from build123d import *

# Parameters (mm, degrees)
SKETCH_1_W          = 76
SKETCH_1_H          = 60
EXTRUDE_1_DEPTH     = 2
EXTRUDE_2_DEPTH     = 3.35
SKETCH_2_W          = 76
SKETCH_2_H          = 60
CUT_EXTRUDE_1_DEPTH = 2.95
SKETCH_3_R          = 2.55
CUT_EXTRUDE_2_DEPTH = 45.193605611
SKETCH_4_R          = 7.5
CUT_EXTRUDE_3_DEPTH = 45.193605611
SKETCH_5_R          = 1.5
CUT_EXTRUDE_4_DEPTH = 45.193605611
SKETCH_6_R          = 2.5
CUT_EXTRUDE_5_DEPTH = 45.193605611
CUT_EXTRUDE_6_DEPTH = 4
CUT_EXTRUDE_7_DEPTH = 4
CUT_EXTRUDE_8_DEPTH = 4


with BuildPart() as part:
    # 草圖1 → 填料-伸長1 (new body)
    with BuildSketch(Plane.XY):
        Rectangle(SKETCH_1_W, SKETCH_1_H)
        with BuildLine():
            ThreePointArc((-6.225922266, -9.22263808), (-5.992959353, -9.526241259), (-6.042909564, -9.905650781))
            Line((-6.042909564, -9.905650781), (-7.592909564, -12.590329533))
            ThreePointArc((-7.592909564, -12.590329533), (-7.896512744, -12.823292446), (-8.275922266, -12.773342235))
            Line((-8.275922266, -12.773342235), (-10.007973074, -11.773342235))
            ThreePointArc((-10.007973074, -11.773342235), (-10.240935987, -11.469739056), (-10.190985776, -11.090329533))
            Line((-10.190985776, -11.090329533), (-8.640985776, -8.405650781))
            ThreePointArc((-8.640985776, -8.405650781), (-8.337382596, -8.172687868), (-7.957973074, -8.22263808))
            Line((-7.957973074, -8.22263808), (-6.225922266, -9.22263808))
        make_face(mode=Mode.SUBTRACT)
        with BuildLine():
            Line((-12.313100093, -5.76593935), (-14.313100093, -9.230040965))
            ThreePointArc((-14.313100093, -9.230040965), (-14.996112795, -9.413053667), (-15.179125497, -8.730040965))
            Line((-15.179125497, -8.730040965), (-13.179125497, -5.26593935))
            ThreePointArc((-13.179125497, -5.26593935), (-12.496112795, -5.082926648), (-12.313100093, -5.76593935))
        make_face(mode=Mode.SUBTRACT)
        with BuildLine():
            ThreePointArc((11.15, -8.780487805), (10.65, -8.280487805), (11.15, -7.780487805))
            Line((11.15, -7.780487805), (15.15, -7.780487805))
            ThreePointArc((15.15, -7.780487805), (15.65, -8.280487805), (15.15, -8.780487805))
            Line((15.15, -8.780487805), (11.15, -8.780487805))
        make_face(mode=Mode.SUBTRACT)
        with BuildLine():
            Line((-5.557090436, 10.186138586), (-7.107090436, 12.870817338))
            ThreePointArc((-7.107090436, 12.870817338), (-7.157040647, 13.250226861), (-6.924077734, 13.55383004))
            Line((-6.924077734, 13.55383004), (-5.192026926, 14.55383004))
            ThreePointArc((-5.192026926, 14.55383004), (-4.812617404, 14.603780251), (-4.509014224, 14.370817338))
            Line((-4.509014224, 14.370817338), (-2.959014224, 11.686138586))
            ThreePointArc((-2.959014224, 11.686138586), (-2.909064013, 11.306729064), (-3.142026926, 11.003125884))
            Line((-3.142026926, 11.003125884), (-4.874077734, 10.003125884))
            ThreePointArc((-4.874077734, 10.003125884), (-5.253487256, 9.953175673), (-5.557090436, 10.186138586))
        make_face(mode=Mode.SUBTRACT)
        with BuildLine():
            Line((1.163100093, 13.546427155), (-0.836899907, 17.01052877))
            ThreePointArc((-0.836899907, 17.01052877), (-0.653887205, 17.693541472), (0.029125497, 17.51052877))
            Line((0.029125497, 17.51052877), (2.029125497, 14.046427155))
            ThreePointArc((2.029125497, 14.046427155), (1.846112795, 13.363414453), (1.163100093, 13.546427155))
        make_face(mode=Mode.SUBTRACT)
    extrude(amount=EXTRUDE_1_DEPTH)

    # 草圖1<3> → 填料-伸長2 (add)
    with BuildSketch(Plane.XY):
        with BuildLine():
            Line((14.7, -0.280487805), (11.6, -0.280487805))
            ThreePointArc((11.6, -0.280487805), (11.246446609, -0.426934414), (11.1, -0.780487805))
            Line((11.1, -0.780487805), (11.1, -2.780487805))
            ThreePointArc((11.1, -2.780487805), (11.246446609, -3.134041195), (11.6, -3.280487805))
            Line((11.6, -3.280487805), (14.7, -3.280487805))
            ThreePointArc((14.7, -3.280487805), (15.053553391, -3.134041195), (15.2, -2.780487805))
            Line((15.2, -2.780487805), (15.2, -0.780487805))
            ThreePointArc((15.2, -0.780487805), (15.053553391, -0.426934414), (14.7, -0.280487805))
        make_face()
        with BuildLine():
            Line((-7.107090436, 12.870817338), (-5.557090436, 10.186138586))
            ThreePointArc((-5.557090436, 10.186138586), (-5.253487256, 9.953175673), (-4.874077734, 10.003125884))
            Line((-4.874077734, 10.003125884), (-3.142026926, 11.003125884))
            ThreePointArc((-3.142026926, 11.003125884), (-2.909064013, 11.306729064), (-2.959014224, 11.686138586))
            Line((-2.959014224, 11.686138586), (-4.509014224, 14.370817338))
            ThreePointArc((-4.509014224, 14.370817338), (-4.812617404, 14.603780251), (-5.192026926, 14.55383004))
            Line((-5.192026926, 14.55383004), (-6.924077734, 13.55383004))
            ThreePointArc((-6.924077734, 13.55383004), (-7.157040647, 13.250226861), (-7.107090436, 12.870817338))
        make_face()
        with BuildLine():
            Line((-6.042909564, -9.905650781), (-7.592909564, -12.590329533))
            ThreePointArc((-7.592909564, -12.590329533), (-7.896512744, -12.823292446), (-8.275922266, -12.773342235))
            Line((-8.275922266, -12.773342235), (-10.007973074, -11.773342235))
            ThreePointArc((-10.007973074, -11.773342235), (-10.240935987, -11.469739056), (-10.190985776, -11.090329533))
            Line((-10.190985776, -11.090329533), (-8.640985776, -8.405650781))
            ThreePointArc((-8.640985776, -8.405650781), (-8.337382596, -8.172687868), (-7.957973074, -8.22263808))
            Line((-7.957973074, -8.22263808), (-6.225922266, -9.22263808))
            ThreePointArc((-6.225922266, -9.22263808), (-5.992959353, -9.526241259), (-6.042909564, -9.905650781))
        make_face()
    extrude(amount=EXTRUDE_2_DEPTH)

    # 草圖2 → 除料-伸長1 (cut)
    with BuildSketch(Plane(origin=(0, 0, 0), x_dir=(-1, 0, 0), z_dir=(0, 0, -1))):
        Rectangle(SKETCH_2_W, SKETCH_2_H)
        with BuildLine():
            ThreePointArc((-29.9, 26.904317068), (-33.435533906, 25.439850974), (-34.9, 21.904317068))
            Line((-34.9, 21.904317068), (-34.9, -21.9))
            ThreePointArc((-34.9, -21.9), (-33.435533906, -25.435533906), (-29.9, -26.9))
            Line((-29.9, -26.9), (29.9, -26.9))
            ThreePointArc((29.9, -26.9), (33.435533906, -25.435533906), (34.9, -21.9))
            Line((34.9, -21.9), (34.9, 21.904317068))
            ThreePointArc((34.9, 21.904317068), (33.435533906, 25.439850974), (29.9, 26.904317068))
            Line((29.9, 26.904317068), (-29.9, 26.904317068))
        make_face(mode=Mode.SUBTRACT)
    extrude(amount=-CUT_EXTRUDE_1_DEPTH, mode=Mode.SUBTRACT)

    # 草圖3 → 除料-伸長2 (cut, through all)
    with BuildSketch(Plane(origin=(0, 0, 0), x_dir=(-1, 0, 0), z_dir=(0, 0, -1))):
        with Locations((20.5, 0)):
            Circle(SKETCH_3_R)
        with Locations((-20.5, 0)):
            Circle(SKETCH_3_R)
        with Locations((-10.25, -17.753520778)):
            Circle(SKETCH_3_R)
        with Locations((-10.25, 17.753520778)):
            Circle(SKETCH_3_R)
        with Locations((10.25, 17.753520778)):
            Circle(SKETCH_3_R)
        with Locations((10.25, -17.753520778)):
            Circle(SKETCH_3_R)
    extrude(amount=-CUT_EXTRUDE_2_DEPTH, mode=Mode.SUBTRACT)

    # 草圖4 → 除料-伸長3 (cut, through all)
    with BuildSketch(Plane(origin=(0, 0, 0), x_dir=(-1, 0, 0), z_dir=(0, 0, -1))):
        Circle(SKETCH_4_R)
    extrude(amount=-CUT_EXTRUDE_3_DEPTH, mode=Mode.SUBTRACT)

    # 草圖5 → 除料-伸長4 (cut, through all)
    with BuildSketch(Plane(origin=(0, 0, 0), x_dir=(-1, 0, 0), z_dir=(0, 0, -1))):
        with Locations((-32.4, 19.404317068)):
            Circle(SKETCH_5_R)
        with Locations(Location((-32.402400032, -19.400309097, 0), (0, 0, 180))):
            Circle(SKETCH_5_R)
        with Locations((32.402400032, -19.400309097)):
            Circle(SKETCH_5_R)
        with Locations((32.402400032, 17.904317068)):
            Circle(SKETCH_5_R)
    extrude(amount=-CUT_EXTRUDE_4_DEPTH, mode=Mode.SUBTRACT)

    # 草圖6 → 除料-伸長5 (cut, through all)
    with BuildSketch(Plane(origin=(0, 0, 0), x_dir=(-1, 0, 0), z_dir=(0, 0, -1))):
        with Locations((-21.9, 16.904317068)):
            Circle(SKETCH_6_R)
        with Locations(Location((21.9, 16.904317068, 0), (0, 0, 180))):
            Circle(SKETCH_6_R)
        with Locations((-21.9, -19.4)):
            Circle(SKETCH_6_R)
    extrude(amount=-CUT_EXTRUDE_5_DEPTH, mode=Mode.SUBTRACT)

    # 草圖7 → 除料-伸長6 (cut)
    with BuildSketch(Plane.ZY.offset(-11.15)):
        Polygon((2, -8.780487805), (0, -8.780487805), (0, -13.780487805), (2, -11.780487805), align=None)
    extrude(amount=-CUT_EXTRUDE_6_DEPTH, mode=Mode.SUBTRACT)

    # 草圖8 → 除料-伸長7 (cut)
    with BuildSketch(Plane(origin=(-5.575, 9.656183252, 0), x_dir=(-0.8660254037844417, -0.4999999999999947, 0), z_dir=(0.49999999999999484, -0.8660254037844418, 0))):
        Polygon((-8.780487805, -2), (-8.780487805, 0), (-13.780487805, 0), (-11.780487805, -2), align=None)
    extrude(amount=-CUT_EXTRUDE_7_DEPTH, mode=Mode.SUBTRACT)

    # 草圖9 → 除料-伸長8 (cut)
    with BuildSketch(Plane(origin=(-5.575, -9.656183252, 0), x_dir=(0.8660254037844359, -0.5000000000000049, 0), z_dir=(0.5000000000000048, 0.8660254037844358, 0))):
        Polygon((-8.780487805, -2), (-8.780487805, 0), (-13.780487805, 0), (-11.780487805, -2), align=None)
    extrude(amount=-CUT_EXTRUDE_8_DEPTH, mode=Mode.SUBTRACT)


solid = part.part
For this review, take the finished solid that the model builds, in its own axes (mm). A direction names the side the tool comes from. Coordinates: 2 decimals unless noted, no trailing zeros. Loops run counter-clockwise (first coordinate to the right, second up) from the corner with the lowest first, then second, coordinate; pieces in that order, holes last. Notation, with made-up numbers: (17.25, 49) - (44.25, 49) arc R28 cw to (44.25, 72) - close; hole circle Ø2 at (58, -25). An arc over 180 degrees is marked (long way). Return JSON: item names as keys, results as strings.
Item 1: For faces 1 (the flat face through (-3.723, 13.01, 2.666)), 2 (the flat face through (13.12, -12.79, 0.99)), 3 (the flat face through (-6.807, -11.229, 2.666)), list the 3-axis set-ups (+Z, -Z, +X, -X, +Y, -Y) from which the entire face can be reached by the end or side of a thin tool; tool diameter is ignored.
Determined:
{"face 1": "+Z, +X, +Y", "face 2": "-Z", "face 3": "+Z, +X, -Y"}
Item 2: Take a section at C-C (x = -21.9). Give the boundary of the cut face in (y, z).
Determined:
{"outline": "(-26.9, 0) - (-2.13, 0) - (-2.13, 2) - (-26.9, 2) - close; (2.13, 0) - (14.4, 0) - (14.4, 2) - (2.13, 2) - close; (19.4, 0) - (26.9, 0) - (26.9, 2) - (19.4, 2) - close"}
Item 3: Mouldability with a two-part tool opening along X and no side actions: class faces 4 (the flat face through (15.2, -2, 3)), 5 (the flat face through (13, -3.28, 3)), 6 (the flat face through (11.1, -2, 3)), 7 (the flat face through (4.519, 17.761, 0.986)) as pulls with the +X half, pulls with the -X half, needs draft (parallel to the pull), parting line crosses it, or undercut.
Determined:
{"face 4": "pulls with the +X half", "face 5": "needs draft", "face 6": "pulls with the -X half", "face 7": "undercut"}
Item 4: Insertion check: pin 1 (4 mm diameter, centred on x = 21.9, y = 16.9, fed in from +Z); pin 2 (6 mm diameter, centred on x = -21.9, y = 16.9, fed in from -Z); pin 3 (6 mm diameter, centred on x = 3, y = -13, fed in from +Z); pin 4 (0.7 mm diameter, centred on y = -2, z = 2.5, fed in from +X). Each pin has a flat end and moves straight along its axis. Give the tip position at first contact, or say it passes through.
Determined:
{"pin 1": "passes through", "pin 2": "stops at z = 0", "pin 3": "stops at z = 2", "pin 4": "stops at x = 15.2"}
Item 5: Take a section at A-A (x = 32.4). Give the boundary of the cut face in (y, z).
Determined:
{"outline": "(-26.23, 0) - (-20.9, 0) - (-20.9, 2) - (-26.23, 2) - close; (-17.9, 0) - (17.9, 0) - (17.9, 2) - (-17.9, 2) - close; (20.9, 0) - (26.23, 0) - (26.23, 2) - (20.9, 2) - close"}
Item 6: Take a section at D-D (z = 0.9). State how many separate pieces and enclosed holes the cut face has, then the cut area to 3 significant figures.
Determined:
{"separate pieces": "1", "enclosed holes": "17", "area": "3,280 mm2"}
Item 7: For line 1 (Y direction, x = -10.25, z = 0.5); line 2 (Y direction, x = 1, z = 1.45); line 3 (X direction, y = -4, z = 0.4), list the stretches that pass through material, from the lowest coordinate up.
Determined:
{"line 1": "y = -26.9 to -20.3, -15.2 to 15.2, 20.3 to 26.9", "line 2": "y = -26.9 to -7.43, 7.43 to 13.83, 18.07 to 26.9", "line 3": "x = -34.9 to -17.76, -15.37 to -6.34, 6.34 to 34.9"}
Item 8: Take a section at B-B (x = 20.5). Give the boundary of the cut face in (y, z), then the cut area to 3 significant figures.
Determined:
{"outline": "(-26.9, 0) - (-21.47, 0) - (-21.47, 2) - (-26.9, 2) - close; (-17.33, 0) - (-2.55, 0) - (-2.55, 2) - (-17.33, 2) - close; (2.55, 0) - (14.83, 0) - (14.83, 2) - (2.55, 2) - close; (18.98, 0) - (26.9, 0) - (26.9, 2) - (18.98, 2) - close", "area": "80.8 mm2"}
